The listing builds one solid part. Answer for the finished solid, in the listing's coordinates (mm). Face numbers are marked on the shaded views. A direction names the side the tool comes from. Round coordinates to 2 decimals unless told otherwise and drop trailing zeros. Loops run counter-clockwise (first coordinate to the right, second up) from the corner with the lowest first, then second, coordinate; pieces in that order, holes last. Notation, with made-up numbers: M 39.25,-27.75 L 60.25,-27.75 A20 ccw 60.25,-2.75 Z; hole C 35.25,67.5 d6. An arc over 180 degrees is marked long. Put each result on its own line as item: value. Start each with the question number.
(1) Section D-D, the plane z = -6.75 is taken. Determine the outline of the cut face in (x, y), then the cut area to 3 significant figures.
(2) Determine the mould class of the marked faces 1, 2, 3 and 4 for opening direction Y: released by +Y, released by -Y, zero draft, split by the parting line, or undercut.
(3) Section A-A, the plane z = 7 is taken. Determine the outline of the cut face in (x, y).
(4) Which of the six approach directions +Z, -Z, +X, -X, +Y, -Y give full straight-line access (tool end or side, diameter ignored) to the marked faces 5, 6, 7 and 8?
(5) Section C-C, the plane y = 0 is taken. Count the separate pieces of the cut face and the enclosed holes in it, then the cut area to 3 significant figures.
(6) Flat-ended cylindrical pins translate along their axes: P1, Ø2, axis at x = -32, y = -8.5, coming from the -Z side; P2, Ø0.6, axis at x = -26, z = -4.5, coming from the +Y side; P3, Ø6, axis at x = -41, z = -7, coming from the -Y side. Find the tip coordinate at first contact, or state that the pin passes through.
(7) Straight lines are drawn through the part: line 1 (X direction, y = 0, z = -5); line 2 (Y direction, x = -35, z = 6.5); line 3 (Z direction, x = -2.2, y = 0). For each, find the intervals that lie inside material, in ascending order.
Autodesk Fusion 360 part; units mm, degrees
sketch "Main Profile" plane through (0, 0, 0) normal (1, 0, 0) x (0, 1, 0)
  line L0 (-19.75, -9.75) -> (19.75, -9.75)
  line L1 (19.75, -9.75) -> (19.75, 9.75)
  line L2 (19.75, 9.75) -> (-19.75, 9.75)
  line L3 (-19.75, 9.75) -> (-19.75, -9.75)
  line L4 (-19.75, -9.75) -> (19.75, 9.75) construction
  line L5 (19.75, -9.75) -> (-19.75, 9.75) construction
  line L6 (-19.75, 3) -> (-25.85, 3)
  line L7 (-25.85, 3) -> (-25.85, -2.8)
  line L8 (-25.85, -2.8) -> (-23.5187, -5.3)
  line L9 (-23.5187, -5.3) -> (-22.05, -5.3)
  line L10 (-22.05, -5.3) -> (-22.05, -3.3)
  line L11 (-22.05, -3.3) -> (-21.35, -3.3)
  line L12 (-21.35, -3.3) -> (-19.75, -4.2238)
  line L13 (0, 9.75) -> (0, -9.75) construction
  line L14 (19.75, 3) -> (25.85, 3)
  line L15 (25.85, 3) -> (25.85, -2.8)
  line L16 (25.85, -2.8) -> (23.5187, -5.3)
  line L17 (23.5187, -5.3) -> (22.05, -5.3)
  line L18 (22.05, -5.3) -> (22.05, -3.3)
  line L19 (22.05, -3.3) -> (21.35, -3.3)
  line L20 (21.35, -3.3) -> (19.75, -4.2238)
  circle A0 centre (0, -0.4) radius 2.75
  dimension "d1" = 39.5
  dimension "d2" = 19.5
  dimension "d3" = 6.1
  dimension "d4" = 6.75
  dimension "d5" = 8.3
  dimension "d6" = 43
  dimension "d7" = 2.5
  dimension "d8" = 120
  dimension "d9" = 3.8
  dimension "d10" = 2
  dimension "d11" = 1.6
  dimension "d12" = 5.5
  dimension "d13" = 0.4
extrude "Extrude1" add sketch "Main Profile" against normal blind 58.25 contours L0 L1 L2 L3 | L3 L6 L7 L8 L9 L10 L11 L12 | L1 L14 L15 L16 L17 L18 L19 L20 | A0
sketch "Side" plane through (0, 0, -9.75) normal (0, 0, -1) x (1, 0, 0)
  line L0 (0, -19.75) -> (0, 19.75)
  line L1 (0, 19.75) -> (-58.25, 19.75)
  line L2 (-58.25, 19.75) -> (-58.25, -19.75)
  line L3 (-58.25, -19.75) -> (0, -19.75)
  circle A0 centre (-35, 0) radius 17.75
  circle A1 centre (-35, 0) radius 7
  line L4 (-10.25, -4.25) -> (-5.75, -4.25)
  line L5 (-5.75, -4.25) -> (-5.75, 4.25)
  line L6 (-5.75, 4.25) -> (-10.25, 4.25)
  line L7 (-10.25, 4.25) -> (-10.25, -4.25)
  line L8 (-10.25, -4.25) -> (-5.75, 4.25) construction
  line L9 (-5.75, -4.25) -> (-10.25, 4.25) construction
  point P0 (-8, 0)
  dimension "d16" = 35.5
  dimension "d17" = 35
  dimension "d18" = 14
  dimension "d19" = 8.5
  dimension "d20" = 4.5
  dimension "d21" = 5.75
extrude "Extrude2" cut sketch "Side" against normal blind 13.5 contours L4 L5 L6 L7
extrude "Extrude3" cut sketch "Side" against normal blind 40 contours A1
extrude "Extrude4" cut sketch "Side" against normal blind 10.85 contours A0
extrude "Extrude5" cut sketch "Main Profile" against normal blind 15.75 contours A0
extrude "Extrude6" cut 1 faces at (-20.8994, 0.8818, 1.1) along direction (0, 0, 1) blind 0.15
chamfer "Chamfer1" distance 1 angle 45 1 edges at (-51.5488, -6.4187, -9.75)
chamfer "Chamfer2" distance 1 angle 45 20 edges at (-58.25, 0, -9.75) (-58.25, -19.75, -6.9869) (-58.25, -20.55, -3.7619) (-58.25, -21.7, -3.3) (-58.25, -22.05, -4.3) (-58.25, -22.7844, -5.3) (-58.25, -24.6844, -4.05) (-58.25, -25.85, 0.1) (-58.25, -22.8, 3) (-58.25, -19.75, 6.375) (-58.25, 0, 9.75) (-58.25, 19.75, 6.375) (-58.25, 22.8, 3) (-58.25, 25.85, 0.1) (-58.25, 24.6844, -4.05) (-58.25, 22.7844, -5.3) (-58.25, 22.05, -4.3) (-58.25, 19.75, -6.9869) (-58.25, 21.7, -3.3) (-58.25, 20.55, -3.7619)
chamfer "Chamfer3" distance 1 angle 45 1 edges at (-41.5263, 2.5313, 1.25)
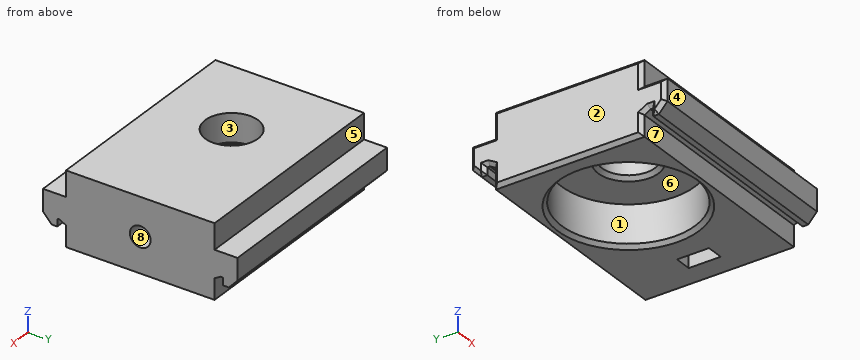
Recorded:
1. outline: M -58.25,-18.75 L -57.25,-19.75 L 0,-19.75 L 0,19.75 L -57.25,19.75 L -58.25,18.75 Z; hole C -35,0 d35.5; hole M -10.25,-4.25 L -5.75,-4.25 L -5.75,4.25 L -10.25,4.25 Z
1. area: 1,270 mm²
2. face 1: undercut
2. face 2: zero draft
2. face 3: undercut
2. face 4: released by -Y
3. outline: M -58.25,-18.75 L -57.25,-19.75 L 0,-19.75 L 0,19.75 L -57.25,19.75 L -58.25,18.75 Z; hole C -35,0 d14
4. face 5: +Z, +X, -X, +Y
4. face 6: -Z
4. face 7: -Z, +X, -X
4. face 8: +X
5. separate pieces: 3
5. enclosed holes: 0
5. area: 501 mm²
6. P1: stops at z = 1.25
6. P2: stops at y = 24.54
6. P3: stops at y = -24.73
7. line 1: x = -58.25 to -52.75, -17.25 to -10.25, -5.75 to 0
7. line 2: y = -19.75 to -7, 7 to 19.75
7. line 3: z = -9.75 to -3.15, 2.35 to 9.75
